Design review of the part built by this model. Coordinates are the model's own, in mm. A direction names the side the tool comes from. Coordinates: 2 decimals unless noted, no trailing zeros. Loops run counter-clockwise (first coordinate to the right, second up) from the corner with the lowest first, then second, coordinate; pieces in that order, holes last. Notation, with made-up numbers: M 11.25,34.25 L 19.25,34.25 A28 cw 19.25,73.25 Z; hole C 46.5,35 d11. An arc over 180 degrees is marked long. Put each result on its own line as item: value. Start each with the question number.
(1) Clearance check with flat-ended pins moving along their axes: pin 1 (3 mm diameter, centred on x = -5.5, y = 4, fed in from +Z); pin 2 (3 mm diameter, centred on x = -5, y = -9, fed in from -Z); pin 3 (4 mm diameter, centred on x = 0, y = -8, fed in from +Z). State where each tip first meets the part, or that it passes through.
(2) Take a section at D-D, the plane x = 5.25. Give the boundary of the cut face in (y, z) (3 decimals), then the cut area to 3 significant figures.
(3) For faces 4 (the flat face through (-3.15, 7, 3)), 5 (the flat face through (-3.15, -14, 3)), 6 (the flat face through (0, 0.375, 3)), 7 (the flat face through (-5, 5, 4.2)), 8 (the flat face through (-5, -9, 4.2)), list the 3-axis set-ups (+Z, -Z, +X, -X, +Y, -Y) from which the entire face can be reached by the end or side of a thin tool; tool diameter is ignored.
(4) For probe 1 along Y at (x, z) = (-5.5, 4.05) (3 decimals); probe 2 along Z at (x, y) = (-0.5, 3); probe 3 along Z at (x, y) = (4, -8), list the stretches that pass through material, from the lowest coordinate up. Write a range as [from, to].
(5) Take a section at B-B, the plane x = 0.5. Give the boundary of the cut face in (y, z) (3 decimals).
(6) The part is to be moulded in two halves that separate along X. For faces 1 (the flat face through (-0.1, -25, 1.7)), 2 (the flat face through (6.75, -8, 2)), 3 (the flat face through (-3.569, 1.896, 3.085)), say which applies: +X half, -X half, draft (parallel to the pull), parting line (faces both ways), or undercut.
(7) Take a section at A-A, the plane y = -12. Give the boundary of the cut face in (x, z), then the cut area to 3 significant figures.
(8) Take a section at C-C, the plane z = 2.45. Give the boundary of the cut face in (x, y) (3 decimals).
```python
from build123d import *

# Parameters (mm, degrees)
F1_DEPTH  = 25
F2_W      = 6.3
F2_H      = 0.75
F3_DEPTH  = 1.5
F4_W      = 3.6
F4_H      = 1
F5_DEPTH  = 0.5
F6_W      = 13.5
F6_H      = 0.25
F7_DEPTH  = 0.2
F8_W      = 13.5
F8_H      = 14.625
F9_DEPTH  = 4.201
F10_R     = 1
F12_DEPTH = 2.701


with BuildPart() as f1:
    # F0 (on Front) → F1 (new body, symmetric)
    with BuildSketch(Plane.XZ):
        Polygon((-6.75, 4.2), (-6.75, 0), (6.75, 0), (6.75, 4.2), (3.15, 4.2), (3.15, 2), (-3.15, 2), (-3.15, 4.2), align=None)
    extrude(amount=F1_DEPTH, both=True)

    # F2 (on face) → F3 (join)
    with BuildSketch(Plane.XY.offset(2)):
        Rectangle(F2_W, F2_H)
    extrude(amount=F3_DEPTH)

    # F4 (on face) → F5 (join)
    with BuildSketch(Plane.XY.offset(4.2)):
        with Locations((4.95, -0.875)):
            Rectangle(F4_W, F4_H)
        with Locations((-4.95, -0.875)):
            Rectangle(F4_W, F4_H)
    extrude(amount=F5_DEPTH)

    # F6 (on face) → F7 (cut)
    with BuildSketch(Plane.XY.offset(4.2)):
        with Locations((0, -6.375)):
            Rectangle(F6_W, F6_H)
        with Locations((0, -11.375)):
            Rectangle(F6_W, F6_H)
        with Locations((0, -16.375)):
            Rectangle(F6_W, F6_H)
    extrude(amount=-F7_DEPTH, mode=Mode.SUBTRACT)

    # F8 (on face) → F9 (cut, through all)
    with BuildSketch(Plane.XY.offset(4.2)):
        with Locations((0, 17.6875)):
            Rectangle(F8_W, F8_H)
    extrude(amount=-F9_DEPTH, mode=Mode.SUBTRACT)

    # F10
    f10_edges = [f1.edges().sort_by_distance(p)[0] for p in [
        (-6.75, 10.375, 2.1),
        (6.75, 10.375, 2.1),
        (-6.75, -25, 2.1),
        (6.75, -25, 2.1),
    ]]
    fillet(f10_edges, radius=F10_R)

    # F11 (on face) → F12 (cut, through all)
    with BuildSketch(Plane.XY.offset(2)):
        Polygon((4, -0.375), (-4, -0.375), (-3.15, -3.375), (3.15, -3.375), align=None)
        Polygon((-3.15, 3.375), (-4, 0.375), (4, 0.375), (3.15, 3.375), align=None)
    extrude(amount=F12_DEPTH, mode=Mode.SUBTRACT)


solid = f1.part
```
Computed values:
1. pin 1: stops at z = 4.2
1. pin 2: stops at z = 0
1. pin 3: stops at z = 2
2. outline: M -25,0 L 10.375,0 L 10.375,4.2 L -0.375,4.2 L -0.375,4.7 L -1.375,4.7 L -1.375,4.2 L -6.25,4.2 L -6.25,4 L -6.5,4 L -6.5,4.2 L -11.25,4.2 L -11.25,4 L -11.5,4 L -11.5,4.2 L -16.25,4.2 L -16.25,4 L -16.5,4 L -16.5,4.2 L -25,4.2 Z
2. area: 149 mm^2
3. face 4: +Z, +Y
3. face 5: +Z, -Y
3. face 6: +Z
3. face 7: +Z, +X, -X, +Y
3. face 8: +Z, +X, -X, -Y
4. probe 1: y = [-25, -16.5], [-16.25, -11.5], [-11.25, -6.5], [-6.25, 10.375]
4. probe 2: z = [0, 2]
4. probe 3: z = [0, 4.2]
5. outline: M -25,0 L 10.375,0 L 10.375,2 L 0.375,2 L 0.375,3.5 L -0.375,3.5 L -0.375,2 L -25,2 Z
6. face 1: draft
6. face 2: +X half
6. face 3: undercut
7. outline: M -6.75,0 L 6.75,0 L 6.75,4.2 L 3.15,4.2 L 3.15,2 L -3.15,2 L -3.15,4.2 L -6.75,4.2 Z
7. area: 42.8 mm^2
8. outline: M -6.75,-24 A1 ccw -5.75,-25 L -3.15,-25 L -3.15,-3.375 L -4,-0.375 L 4,-0.375 L 3.15,-3.375 L 3.15,-25 L 5.75,-25 A1 ccw 6.75,-24 L 6.75,9.375 A1 ccw 5.75,10.375 L 3.15,10.375 L 3.15,3.375 L 4,0.375 L -4,0.375 L -3.15,3.375 L -3.15,10.375 L -5.75,10.375 A1 ccw -6.75,9.375 Z
